```python
from build123d import *

# Parameters (mm, degrees)
F0_W      = 67
F0_H      = 50
F1_DEPTH  = 70
F2_W      = 29
F2_H      = 3.3
F3_DEPTH  = 67.001
F4_R      = 3.15
F5_DEPTH  = 12.5
F7_DEPTH  = 1.5
F9_DEPTH  = 67.001
F11_R     = 20
F12_DEPTH = 1.5
F14_R     = 20
F15_DEPTH = 1.5


with BuildPart() as f1:
    # F0 (on Top) → F1 (new body)
    with BuildSketch(Plane.XY):
        with Locations((33.5, 25)):
            Rectangle(F0_W, F0_H)
    extrude(amount=F1_DEPTH)

    # F2 (on face) → F3 (cut, through all)
    with BuildSketch(Plane.YZ.offset(67)):
        with Locations((35.5, 55.85)):
            Rectangle(F2_W, F2_H)
    extrude(amount=-F3_DEPTH, mode=Mode.SUBTRACT)

    # F4 (on face) → F5 (cut, through all)
    with BuildSketch(Plane.XY.offset(70)):
        with Locations((33.5, 41.7)):
            Circle(F4_R)
    extrude(amount=-F5_DEPTH, mode=Mode.SUBTRACT)

    # F6 (on face) → F7 (cut)
    with BuildSketch(Plane.XZ):
        Polygon((0, 6.9418640507), (0, 0), (30.1778222043, 31.5290679747), (26.8556444086, 35), align=None)
        Polygon((30.1778222043, 31.5290679747), (0, 0), (6.6443555914, 0), (33.5, 28.0581359493), align=None)
        Polygon((26.8556444086, 35), (30.1778222043, 31.5290679747), (33.5, 35), (30.1778222043, 38.4709320253), align=None)
        Polygon((33.5, 35), (30.1778222043, 31.5290679747), (33.5, 28.0581359493), (36.8221777957, 31.5290679747), align=None)
        Polygon((30.1778222043, 38.4709320253), (33.5, 35), (36.8221777957, 38.4709320253), (33.5, 41.9418640507), align=None)
        Polygon((36.8221777957, 38.4709320253), (33.5, 35), (36.8221777957, 31.5290679747), (40.1443555914, 35), align=None)
        Polygon((0, 63.0581359493), (26.8556444086, 35), (30.1778222043, 38.4709320253), (0, 70), align=None)
        Polygon((36.8221777957, 31.5290679747), (33.5, 28.0581359493), (60.3556444086, 0), (67, 0), align=None)
        Polygon((33.5, 41.9418640507), (36.8221777957, 38.4709320253), (67, 70), (60.3556444086, 70), align=None)
        Polygon((67, 70), (36.8221777957, 38.4709320253), (40.1443555914, 35), (67, 63.0581359493), align=None)
        Polygon((0, 70), (30.1778222043, 38.4709320253), (33.5, 41.9418640507), (6.6443555914, 70), align=None)
        Polygon((40.1443555914, 35), (36.8221777957, 31.5290679747), (67, 0), (67, 6.9418640507), align=None)
    extrude(amount=-F7_DEPTH, mode=Mode.SUBTRACT)

    # F8 (on face) → F9 (cut, through all)
    with BuildSketch(Plane.YZ.offset(67)):
        with BuildLine():
            Line((43.4544826719, 36.5), (10.5455173281, 36.5))
            ThreePointArc((10.5455173281, 36.5), (8, 27), (10.5455173281, 17.5))
            Line((10.5455173281, 17.5), (43.4544826719, 17.5))
            ThreePointArc((43.4544826719, 17.5), (45.3525906995, 22.0824381431), (46, 27))
            ThreePointArc((46, 27), (45.3525906995, 31.9175618569), (43.4544826719, 36.5))
        make_face()
        with BuildLine():
            ThreePointArc((43.4544826719, 36.5), (27, 46), (10.5455173281, 36.5))
            Line((10.5455173281, 36.5), (43.4544826719, 36.5))
        make_face()
        with BuildLine():
            Line((43.4544826719, 17.5), (10.5455173281, 17.5))
            ThreePointArc((10.5455173281, 17.5), (27, 8), (43.4544826719, 17.5))
        make_face()
        with BuildLine():
            Line((50, 36.5), (43.4544826719, 36.5))
            ThreePointArc((43.4544826719, 36.5), (45.3525906995, 31.9175618569), (46, 27))
            Line((46, 27), (50, 27))
            Line((50, 27), (50, 36.5))
        make_face()
        with BuildLine():
            ThreePointArc((46, 27), (45.3525906995, 22.0824381431), (43.4544826719, 17.5))
            Line((43.4544826719, 17.5), (50, 17.5))
            Line((50, 17.5), (50, 27))
            Line((50, 27), (46, 27))
        make_face()
    extrude(amount=-F9_DEPTH, mode=Mode.SUBTRACT)

    # F11 (on offset) → F12 (cut)
    with BuildSketch(Plane.YZ.offset(56)):
        with Locations((27, 27)):
            Circle(F11_R)
    extrude(amount=-F12_DEPTH, mode=Mode.SUBTRACT)

    # F14 (on offset) → F15 (cut)
    with BuildSketch(Plane.YZ.offset(12.5)):
        with Locations((27, 27)):
            Circle(F14_R)
    extrude(amount=-F15_DEPTH, mode=Mode.SUBTRACT)


solid = f1.part
```
Verification items for the finished model (mm, model axes). A direction names the side the tool comes from. Give positions to 0.01 mm unless a question says otherwise; leave off trailing zeros. Loops run counter-clockwise (first coordinate to the right, second up) from the corner with the lowest first, then second, coordinate; pieces in that order, holes last.
1. Section check B-B, the plane y = 18.5. Enter the section's corners in (x, z).
2. Section check A-A, the plane y = 27. Enter the section's corners in (x, z), then the cut area to 3 significant figures.
3. Set-up check for faces 1 (the flat face through (33, 1.5, 38)), 2 (the flat face through (34, 35, 54.2)), 3 (the flat face through (54.5, 7.6, 27.1)): record each of +Z, -Z, +X, -X, +Y, -Y from which the full face is reachable in a straight line by a thin tool's end or side.
4. Section check C-C, the plane x = 32.5. Enter the section's corners in (y, z), then the cut area to 3 significant figures.
5. Section check D-D, the plane z = 27. Enter the section's corners in (x, y), then the cut area to 3 significant figures.
6. Mould release check, pull along X, two halves, no side actions. Record for faces 4 (the cylindrical face through (11.76, 7.014, 27.741)), 5 (the flat face through (10, 0, 35)), 6 (the flat face through (0, 14, 42)): released by +X, released by -X, zero draft, split by the parting line, or undercut.
7. Thickness scan on line 1 (Z direction, x = 11.7, y = 27); line 2 (Z direction, x = 31.5, y = 47.5); line 3 (X direction, y = 22.5, z = 45.5). Record the ranges inside material, lowest first.
8. Go/stop test with flat-tipped pins: pin 1 Ø1 at (x, z) = (22.5, 26.5) entering from -Y; pin 2 Ø19 at (y, z) = (29, 26) entering from +X; pin 3 Ø1.6 at (x, z) = (23.5, 55.5) entering from +Y. Record where each tip stops, or that it passes through.
Geometry says:
1. outline: (0, 0) - (67, 0) - (67, 10.01) - (56, 10.01) - (56, 8.9) - (54.5, 8.9) - (54.5, 10.01) - (12.5, 10.01) - (12.5, 8.9) - (11, 8.9) - (11, 10.01) - (0, 10.01) - close; (0, 43.99) - (11, 43.99) - (11, 45.1) - (12.5, 45.1) - (12.5, 43.99) - (54.5, 43.99) - (54.5, 45.1) - (56, 45.1) - (56, 43.99) - (67, 43.99) - (67, 70) - (0, 70) - close
2. outline: (0, 0) - (67, 0) - (67, 8) - (56, 8) - (56, 7) - (54.5, 7) - (54.5, 8) - (12.5, 8) - (12.5, 7) - (11, 7) - (11, 8) - (0, 8) - close; (0, 46) - (11, 46) - (11, 47) - (12.5, 47) - (12.5, 46) - (54.5, 46) - (54.5, 47) - (56, 47) - (56, 46) - (67, 46) - (67, 54.2) - (0, 54.2) - close; (0, 57.5) - (67, 57.5) - (67, 70) - (0, 70) - close
2. area: 1,920 mm2
3. face 1: -Y
3. face 2: +X, -X, +Y
3. face 3: none
4. outline: (0, 0) - (50, 0) - (50, 17.5) - (43.45, 17.5) arc R19 cw (long way) to (43.45, 36.5) - (50, 36.5) - (50, 54.2) - (21, 54.2) - (21, 57.5) - (38.71, 57.5) - (38.71, 70) - (0, 70) - (0, 42.99) - (1.5, 42.99) - (1.5, 27.01) - (0, 27.01) - close; (44.69, 57.5) - (50, 57.5) - (50, 70) - (44.69, 70) - close
4. area: 2,080 mm2
5. outline: (0, 0) - (19.2, 0) - (19.2, 1.5) - (32.49, 1.5) - (32.49, 0) - (34.51, 0) - (34.51, 1.5) - (47.8, 1.5) - (47.8, 0) - (67, 0) - (67, 8) - (56, 8) - (56, 7) - (54.5, 7) - (54.5, 8) - (12.5, 8) - (12.5, 7) - (11, 7) - (11, 8) - (0, 8) - close
5. area: 493 mm2
6. face 4: undercut
6. face 5: zero draft
6. face 6: released by -X
7. line 1: z = 0 to 7, 47 to 54.2, 57.5 to 70
7. line 2: z = 0 to 17.5, 36.5 to 54.2, 57.5 to 70
7. line 3: x = 0 to 11, 12.5 to 54.5, 56 to 67
8. pin 1: stops at y = 1.5
8. pin 2: passes through
8. pin 3: stops at y = 21
